The listing builds one solid part. Answer for the finished solid, in the listing's coordinates (mm). Coordinates: 2 decimals unless noted, no trailing zeros. Write each loop counter-clockwise with the first axis right and the second up, starting at its lowest first coordinate (ties: lowest second). Pieces come first, ordered by that corner, then holes.
from build123d import *

# Parameters (mm, degrees)
EXTRUDE_1_DEPTH = 83


with BuildPart() as part:
    # 草图1 → 凸台-拉伸1 (new body)
    with BuildSketch(Plane.XY):
        with BuildLine():
            ThreePointArc((42.5, 59.659974019), (22.309968658, 69.769820112), (0, 73.25))
            ThreePointArc((0, 73.25), (-22.309968658, 69.769820112), (-42.5, 59.659974019))
            Line((-42.5, 59.659974019), (-42.5, -59.659974019))
            ThreePointArc((-42.5, -59.659974019), (-22.309968513, -69.769820159), (3.06e-07, -73.25))
            ThreePointArc((3.06e-07, -73.25), (22.309968804, -69.769820065), (42.5, -59.659974019))
            Line((42.5, -59.659974019), (42.5, 59.659974019))
        make_face()
        with BuildLine():
            Line((42.5, -73.25), (42.5, -59.659974019))
            ThreePointArc((42.5, -59.659974019), (22.309968804, -69.769820065), (3.06e-07, -73.25))
            Line((3.06e-07, -73.25), (42.5, -73.25))
        make_face()
        with BuildLine():
            ThreePointArc((3.06e-07, -73.25), (-22.309968513, -69.769820159), (-42.5, -59.659974019))
            Line((-42.5, -59.659974019), (-42.5, -73.25))
            Line((-42.5, -73.25), (3.06e-07, -73.25))
        make_face()
    extrude(amount=EXTRUDE_1_DEPTH)


solid = part.part
1. Section A-A on z = 41 is taken. Give the vertices of the cut face in (x, y), then the cut area to 3 significant figures.
Results found:
outline: (-42.5, -73.25) - (42.5, -73.25) - (42.5, 59.66) arc R73.25 ccw to (-42.5, 59.66) - close
area: 12,100 mm2
2. Section B-B on x = 24 is taken. Give the vertices of the cut face in (y, z), then the cut area to 3 significant figures.
Results found:
outline: (-73.25, 0) - (69.21, 0) - (69.21, 83) - (-73.25, 83) - close
area: 11,800 mm2
3. Section C-C on x = 34.5 is taken. Give the vertices of the cut face in (y, z).
Results found:
outline: (-73.25, 0) - (64.62, 0) - (64.62, 83) - (-73.25, 83) - close
4. A flat-ended cylindrical pin translates along its axis: P1, Ø3, axis at x = 22.5, z = 56, coming from the +Y side. Find the tip coordinate at first contact, or state that the pin passes through.
Results found:
P1: stops at y = 70.18
5. Find the intervals of material crossed by L1, parallel to Y at x = 1, z = 42; L2, parallel to Y at x = 38, z = 44.5; L3, parallel to X at y = 65, z = 65.5, in increasing order.
Results found:
L1: y = -73.25 to 73.24
L2: y = -73.25 to 62.62
L3: x = -33.77 to 33.77
